Print and shaded views of the part. All mm, measured from the part's lowest x, y and z. Coordinates: 2 decimals unless noted, no trailing zeros. Order: outer loops, then holes, each group sorted by start corner. A loop starts at its lowest first (then second) coordinate and runs counter-clockwise, first axis right, second up. Notation, with made-up numbers: M -1,56 L 54,56 A25 cw 54,78 Z; hole C 63,-1.5 d3. An arc over 180 degrees is marked long. Return JSON: item names as keys, results as strings.
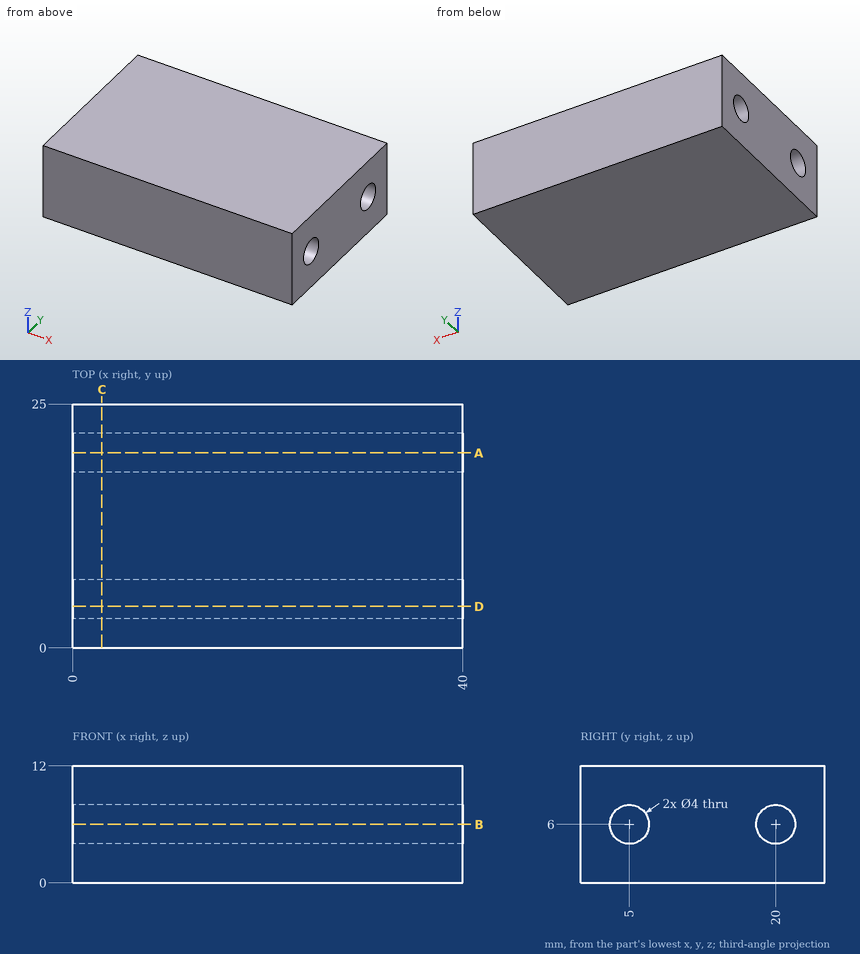
Item 1: Wall check: line 1 (Y direction, x = 10.5, z = 6); line 2 (Y direction, x = 16, z = 4.25); line 3 (Z direction, x = 26, y = 5.75). Give the ranges that are in metal, low to high.
Check result:
{"line 1": "y = 0 to 3, 7 to 18, 22 to 25", "line 2": "y = 0 to 4.03, 5.97 to 19.03, 20.97 to 25", "line 3": "z = 0 to 4.15, 7.85 to 12"}
Item 2: Saw through at D-D (y = 4.25). Write the cut outline in (x, z).
Check result:
{"outline": "M 0,0 L 40,0 L 40,4.15 L 0,4.15 Z; M 0,7.85 L 40,7.85 L 40,12 L 0,12 Z"}
Item 3: Saw through at A-A (y = 20). Write the cut outline in (x, z).
Check result:
{"outline": "M 0,0 L 40,0 L 40,4 L 0,4 Z; M 0,8 L 40,8 L 40,12 L 0,12 Z"}
Item 4: Saw through at C-C (x = 3). Write the cut outline in (y, z).
Check result:
{"outline": "M 0,0 L 25,0 L 25,12 L 0,12 Z; hole C 5,6 d4; hole C 20,6 d4"}
Item 5: Saw through at B-B (z = 6). Write the cut outline in (x, y).
Check result:
{"outline": "M 0,0 L 40,0 L 40,3 L 0,3 Z; M 0,7 L 40,7 L 40,18 L 0,18 Z; M 0,22 L 40,22 L 40,25 L 0,25 Z"}
Item 6: Drop a flat-ended pin along its axis: pin 1 Ø12 at (x, y) = (14.5, 11.5) entering from -Z. Give the stop position or say it passes through.
Check result:
{"pin 1": "stops at z = 0"}
